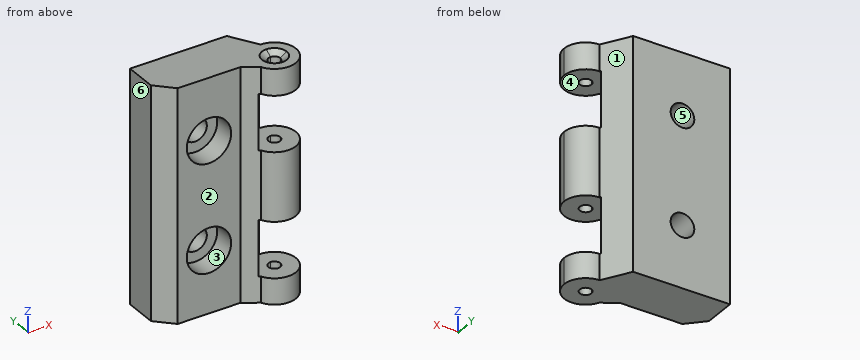
from build123d import *

# Parameters (mm, degrees)
F1_DEPTH       = 43
F2_T1_DEPTH    = 43
F2_T3_DEPTH    = 58.4300979278
F4_D           = 4.4
F4_CBORE_D     = 8.25
F4_CBORE_DEPTH = 4
F5_SIZE2       = 4.99999
F5_SIZE        = 2.99999
F7_START       = 4.8
F6_R           = 4.2
F7_DEPTH       = 10.3
F8_START       = 27.8
F8_DEPTH       = 10.3
F9_SIZE2       = 1.2
F9_SIZE        = 0.8


# Not quite as in the source:
# - a fillet or chamfer that OpenCascade refuses, or shapes differently, is made with other operations: its cross-section is extruded or revolved along the edge and cut away or added
# - a fillet or chamfer is up to 0.001 mm smaller than in the source, because OpenCascade refuses the exact size


with BuildPart() as f1:
    # F0 (on Top) → F1 (new body)
    with BuildSketch(Plane.XY):
        with BuildLine():
            Line((-10.5, -4.5), (6.5, -4.5))
            ThreePointArc((6.5, -4.5), (7.6715728753, -1.6715728753), (10.5, -0.5))
            Line((10.5, -0.5), (10.5, 4.5))
            Line((10.5, 4.5), (-10.5, 4.5))
            Line((-10.5, 4.5), (-10.5, -4.5))
        make_face()
        with BuildLine():
            Line((6.5, -4.5), (9.4, -4.5))
            ThreePointArc((9.4, -4.5), (9.7221825407, -3.7221825407), (10.5, -3.4))
            Line((10.5, -3.4), (10.5, -0.5))
            ThreePointArc((10.5, -0.5), (7.6715728753, -1.6715728753), (6.5, -4.5))
        make_face()
        with BuildLine():
            ThreePointArc((11.6, -4.5), (10.5, -5.6), (9.4, -4.5))
            Line((9.4, -4.5), (6.5, -4.5))
            ThreePointArc((6.5, -4.5), (10.5, -8.5), (14.5, -4.5))
            ThreePointArc((14.5, -4.5), (13.3284271247, -1.6715728753), (10.5, -0.5))
            Line((10.5, -0.5), (10.5, -3.4))
            ThreePointArc((10.5, -3.4), (11.2778174593, -3.7221825407), (11.6, -4.5))
        make_face()
    extrude(amount=F1_DEPTH)

    # F2: chamfer of 3 on 2 edges, made by hand

    # F2_s2 → F2_t1 (join)
    with BuildSketch(Plane.XY):
        with BuildLine():
            Line((4.1754446797, -4.5), (6.8859683884, -6.2142857143))
            ThreePointArc((6.8859683884, -6.2142857143), (6.6075772395, -5.4214364079), (6.5, -4.5))
            Line((6.5, -4.5), (4.1754446797, -4.5))
        make_face()
    extrude(amount=F2_T1_DEPTH)

    # F2_s4 → F2_t3 (cut)
    with BuildSketch(Plane.XY.offset(-7.7150489639)):
        Polygon((-7.5, -4.5), (-10.5, -1.5), (-10.5, -4.5), align=None)
    extrude(amount=F2_T3_DEPTH, mode=Mode.SUBTRACT)

    # F4 (through all)
    with Locations(Plane.XZ.offset(4.5)):
        with Locations((-1.6622776602, 31.5), (-1.6622776602, 11.5)):
            CounterBoreHole(F4_D / 2, F4_CBORE_D / 2, F4_CBORE_DEPTH)

    # F5 (size 3 and 5 in the source; OpenCascade refuses exactly that, so slightly less here)
    f5_edges = [f1.edges().sort_by_distance(p)[0] for p in [
        (10.5, 4.5, 21.5),
    ]]
    f5_side = f1.faces().sort_by_distance((0.057932, 4.5, 21.5))[0]
    chamfer(f5_edges, length=F5_SIZE, length2=F5_SIZE2, reference=f5_side)

    # F6 (on face) → F7 (cut)
    with BuildSketch(Plane.XY.offset(F7_START)):
        with Locations((10.5, -4.5)):
            Circle(F6_R)
    extrude(amount=F7_DEPTH, mode=Mode.SUBTRACT)

    # F6 (on face) → F8 (cut)
    with BuildSketch(Plane.XY.offset(F8_START)):
        with Locations((10.5, -4.5)):
            Circle(F6_R)
    extrude(amount=F8_DEPTH, mode=Mode.SUBTRACT)

    # F9
    f9_edges = [f1.edges().sort_by_distance(p)[0] for p in [
        (10.5, -5.6, 43),
    ]]
    f9_side = f1.faces().sort_by_distance((10.5, -5.6, 40.55))[0]
    chamfer(f9_edges, length=F9_SIZE, length2=F9_SIZE2, reference=f9_side)


solid = f1.part
Part model, mm, in its own coordinate system. Face numbers are marked on the shaded views. A direction names the side the tool comes from. Coordinates: 2 decimals unless noted, no trailing zeros. Order: outer loops, then holes, each group sorted by start corner. A loop starts at its lowest first (then second) coordinate and runs counter-clockwise, first axis right, second up. Notation, with made-up numbers: M 16,84.25 L 69,84.25 A16 cw 69,105.25 Z; hole C 6,55 d6. An arc over 180 degrees is marked long. One line per question, with ' | ' between items.
Q1. Pin check, flat tips, straight feed: P1, Ø1.5, axis at x = -5.5, z = 28.5, coming from the -Y side; P2, Ø2.5, axis at x = -2, z = 9.5, coming from the -Y side; P3, Ø5, axis at x = 10, z = 11.5, coming from the -Y side. Stop position of each tip, or through.
A:
P1: stops at y = -4.5 | P2: stops at y = -0.5 | P3: stops at y = -1.56
Q2. 3-axis set-ups, long thin cutter, end or side, ignore diameter. For the marked faces 1, 2 and 3: which of +Z, -Z, +X, -X, +Y, -Y reach the whole face in a straight line?
A:
face 1: +Z, -Z, +X, +Y | face 2: +Z, -Z, -X, -Y | face 3: -Y
Q3. Slice it at B-B (y = -7.5). Give the cut face in (x, z), and give its area (3 significant figures).
A:
outline: M 7.85,0 L 13.15,0 L 13.15,4.8 L 7.85,4.8 Z; M 7.85,15.1 L 13.15,15.1 L 13.15,27.8 L 7.85,27.8 Z; M 7.85,38.1 L 13.15,38.1 L 13.15,43 L 7.85,43 Z | area: 119 mm^2
Q4. Slice it at C-C (y = 3.25). Give the cut face in (x, z), and give its area (3 significant figures).
A:
outline: M -10.5,0 L 8.25,0 L 8.25,43 L -10.5,43 Z; hole C -1.66,11.5 d4.4; hole C -1.66,31.5 d4.4 | area: 776 mm^2
Q5. Two-plate mould, pull along X, no slides. Class the marked faces 4, 5 and 6: +X half, -X half, draft (parallel to the pull), parting line (faces both ways), or undercut.
A:
face 4: draft | face 5: undercut | face 6: -X half
Q6. Drill centre lines: line 1 (Z direction, x = 12.25, y = -6.75); line 2 (Z direction, x = 9.5, y = -3.75); line 3 (Y direction, x = 2.5, z = 18.5). Where is each one in solid material? Low to high.
A:
line 1: z = 0 to 4.8, 15.1 to 27.8, 38.1 to 43 | line 2: z = 0 to 4.8, 15.1 to 27.8, 38.1 to 42.3 | line 3: y = -4.5 to 4.5
Q7. Slice it at D-D (z = 11.5). Give the cut face in (x, y).
A:
outline: M -10.5,-1.5 L -7.5,-4.5 L -5.79,-4.5 L -5.79,-0.5 L -3.86,-0.5 L -3.86,4.5 L -10.5,4.5 Z; M 0.54,-0.5 L 2.46,-0.5 L 2.46,-4.5 L 4.18,-4.5 L 6.59,-6.02 A4.2 cw 10.38,-0.3 L 7.5,4.5 L 0.54,4.5 Z
